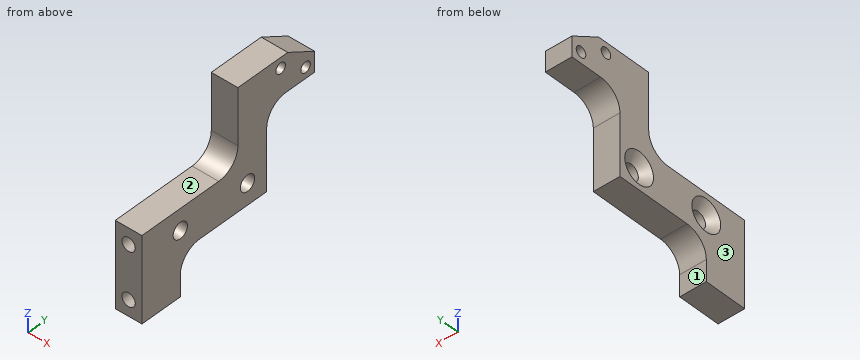
from build123d import *

# Parameters (mm, degrees)
SKETCH1_R                       = 1.5
SKETCH1_R_2                     = 1
BOSS_EXTRUDE1_DEPTH             = 5
FILLET1_R                       = 4
TAP_DRILL_FOR_M3X0_5_TAP1_D     = 2.5
TAP_DRILL_FOR_M3X0_5_TAP1_DEPTH = 4
CHAMFER1_SIZE                   = 1.5


with BuildPart() as part:
    # Sketch1 → Boss-Extrude1 (new body)
    with BuildSketch(Plane(origin=(0, 0, 0), x_dir=(0, 0, -1), z_dir=(1, 0, 0))):
        Polygon((30.5, 0), (14.5, 0), (14.5, 20), (0, 20), (0, 30.4), (3.233161507, 36), (7, 36), (7, 26), (22.5, 26), (22.5, 8), (30.5, 8), align=None)
        with Locations((18.5, 8)):
            Circle(SKETCH1_R, mode=Mode.SUBTRACT)
        with Locations((18.5, 22)):
            Circle(SKETCH1_R, mode=Mode.SUBTRACT)
        with Locations((1.95, 28.91)):
            Circle(SKETCH1_R_2, mode=Mode.SUBTRACT)
        with Locations((4.95, 34.106152423)):
            Circle(SKETCH1_R_2, mode=Mode.SUBTRACT)
    extrude(amount=BOSS_EXTRUDE1_DEPTH)

    # Fillet1
    fillet1_edges = [part.edges().sort_by_distance(p)[0] for p in [
        (2.5, 20, -14.5),
        (2.5, 26, -7),
        (2.5, 8, -22.5),
    ]]
    fillet(fillet1_edges, radius=FILLET1_R)

    # Tap Drill for M3x0.5 Tap1
    with Locations(Plane(origin=(0, 0, 0), x_dir=(-1, 0, 0), z_dir=(0, -1, 0))):
        with Locations((-2.5, 17.5), (-2.5, 27.5)):
            Hole(TAP_DRILL_FOR_M3X0_5_TAP1_D / 2, depth=TAP_DRILL_FOR_M3X0_5_TAP1_DEPTH)

    # Chamfer1
    chamfer1_edges = [part.edges().sort_by_distance(p)[0] for p in [
        (0, 8, -17),
        (0, 22, -17),
    ]]
    chamfer(chamfer1_edges, length=CHAMFER1_SIZE)


solid = part.part
Verification items for the finished model (mm, model axes). Face numbers are marked on the shaded views. A direction names the side the tool comes from. Coordinates: 2 decimals unless noted, no trailing zeros. Order: outer loops, then holes, each group sorted by start corner. A loop starts at its lowest first (then second) coordinate and runs counter-clockwise, first axis right, second up.
1. Sectioned sample at A-A, the plane y = 22. Record the cut outline in (x, z).
Results found:
outline: (0, -22.5) - (5, -22.5) - (5, -20) - (1.5, -20) - (0, -21.5) - close; (0, -15.5) - (1.5, -17) - (5, -17) - (5, 0) - (0, 0) - close
2. Go/stop test with flat-tipped pins: pin 1 Ø2.5 at (y, z) = (8, -18.5) entering from +X (3 decimals); pin 2 Ø2.5 at (x, z) = (2, -19.5) entering from +Y; pin 3 Ø2.5 at (x, y) = (2.5, 34) entering from -Z; pin 4 Ø5 at (y, z) = (22, -18.5) entering from -X. Record where each tip stops, or that it passes through.
Results found:
pin 1: passes through
pin 2: stops at y = 26
pin 3: stops at z = -7
pin 4: stops at x = 0.5
3. Set-up check for the marked faces 1, 2 and 3: record each of +Z, -Z, +X, -X, +Y, -Y from which the full face is reachable in a straight line by a thin tool's end or side.
Results found:
face 1: -Z, +X, -X, +Y
face 2: +Z, +X, -X, -Y
face 3: +Z, -Z, -X, +Y, -Y
4. Sectioned sample at C-C, the plane x = 2.5. Record the cut outline in (y, z).
Results found:
outline: (0, -30.5) - (8, -30.5) - (8, -26.5) arc R4 cw to (12, -22.5) - (26, -22.5) - (26, -11) arc R4 cw to (30, -7) - (36, -7) - (36, -3.23) - (30.4, 0) - (20, 0) - (20, -10.5) arc R4 cw to (16, -14.5) - (0, -14.5) - (0, -16.25) - (4, -16.25) - (4, -18.75) - (0, -18.75) - (0, -26.25) - (4, -26.25) - (4, -28.75) - (0, -28.75) - close; hole circle Ø3 at (8, -18.5); hole circle Ø3 at (22, -18.5); hole circle Ø2 at (28.91, -1.95); hole circle Ø2 at (34.11, -4.95)
5. Scan lines: line 1 (Z direction, x = 2.5, y = 3.05); line 2 (Y direction, x = 3.2, z = -4.95); line 3 (Y direction, x = 2.2, z = -26.5). Record each from-to range of solid material in increasing order.
Results found:
line 1: z = -30.5 to -28.75, -26.25 to -18.75, -16.25 to -14.5
line 2: y = 20 to 33.11, 35.11 to 36
line 3: y = 4 to 8
6. Sectioned sample at D-D, the plane z = -27.5. Record the cut outline in (x, y).
Results found:
outline: (0, 0) - (1.25, 0) - (1.25, 4) - (3.75, 4) - (3.75, 0) - (5, 0) - (5, 8) - (0, 8) - close
7. Sectioned sample at B-B, the plane z = -4.95. Record the cut outline in (x, y).
Results found:
outline: (0, 20) - (5, 20) - (5, 33.11) - (0, 33.11) - close; (0, 35.11) - (5, 35.11) - (5, 36) - (0, 36) - close
